Verification items for the finished model (mm, model axes). Face numbers are marked on the shaded views. A direction names the side the tool comes from. Round coordinates to 2 decimals unless told otherwise and drop trailing zeros. Loops run counter-clockwise (first coordinate to the right, second up) from the corner with the lowest first, then second, coordinate; pieces in that order, holes last. Notation, with made-up numbers: M 0,15.5 L 31,15.5 A27 ccw 31,52.5 Z; hole C -18,81 d1. An arc over 180 degrees is marked long. Write item = value, one per line. Start each with the question number.
from build123d import *

# Parameters (mm, degrees)
SKETCH_R     = 4
PAD_DEPTH    = 13
SKETCH001_R  = 2.5
POCKET_DEPTH = 5
FILLET_R     = 14


with BuildPart() as part:
    # Sketch → Pad (new body)
    with BuildSketch(Plane.XY):
        Polygon((27.5, 0), (-27.5, 0), (-27.5, 5), (-14.5, 5), (-14.5, 29), (14.5, 29), (14.5, 5), (27.5, 5), align=None)
        with Locations((0, 14.5)):
            Circle(SKETCH_R, mode=Mode.SUBTRACT)
    extrude(amount=PAD_DEPTH)

    # Sketch001 → Pocket (cut)
    with BuildSketch(Plane.XZ):
        with Locations((-21, 6.5)):
            Circle(SKETCH001_R)
        with Locations((21, 6.5)):
            Circle(SKETCH001_R)
    extrude(amount=-POCKET_DEPTH, mode=Mode.SUBTRACT)

    # Fillet
    fillet_edges = [part.edges().sort_by_distance(p)[0] for p in [
        (-14.5, 29, 6.5),
        (14.5, 29, 6.5),
    ]]
    fillet(fillet_edges, radius=FILLET_R)


solid = part.part
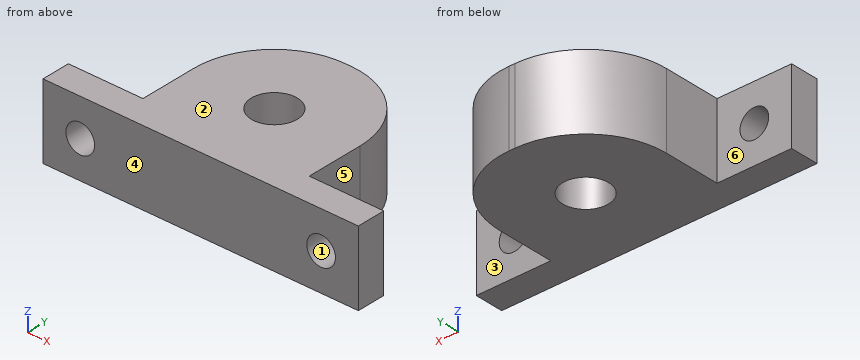
1. Thickness scan on line 1 (X direction, y = 14.25, z = 9.25); line 2 (Z direction, x = 21, y = 2.5); line 3 (Y direction, x = 0, z = 7). Record the ranges inside material, lowest first.
2. Mould release check, pull along Z, two halves, no side actions. Record for the marked faces 1, 2 and 3: pulls with the +Z half, pulls with the -Z half, needs draft (parallel to the pull), parting line crosses it, or undercut.
3. Tool access check on the marked faces 4, 5 and 6. Record the directions out of +Z, -Z, +X, -X, +Y, -Y that give a thin tool (end or side, any length) a straight path to the whole face; none if there is none.
4. Section check B-B, the plane x = 21. Enter the section's corners in (y, z).
5. Gauge pin test, flat ends, axial feed: P1, Ø4.5, axis at x = 21, z = 6.5, coming from the -Y side; P2, Ø1, axis at x = 13.5, z = 9.5, coming from the +Y side; P3, Ø4, axis at y = 24.5, z = 11, coming from the +X side; P4, Ø3, axis at y = 8, z = 3, coming from the +X side. Record the tip position at first contact, or that the pin passes through.
6. Section check D-D, the plane x = 2. Enter the section's corners in (y, z).
7. Section check C-C, the plane x = -16. Enter the section's corners in (y, z), and give its area (3 significant figures).
8. Section check A-A, the plane z = 6.5. Enter the section's corners in (x, y), and give its area (3 significant figures).
Computed values:
q1.line_1 = -14.5 to -3.99, 3.99 to 14.5
q1.line_2 = 0 to 4, 9 to 13
q1.line_3 = 0 to 10.5, 18.5 to 29
q2.face_1 = undercut
q2.face_2 = pulls with the +Z half
q2.face_3 = needs draft
q3.face_4 = +Z, -Z, +X, -X, -Y
q3.face_5 = +Z, -Z, +X, +Y
q3.face_6 = +Z, -Z, -X, +Y
q4.outline = M 0,0 L 5,0 L 5,4 L 0,4 Z; M 0,9 L 5,9 L 5,13 L 0,13 Z
q5.P1 = through
q5.P2 = 21.3
q5.P3 = 12.32
q5.P4 = 14.5
q6.outline = M 0,0 L 11.04,0 L 11.04,13 L 0,13 Z; M 17.96,0 L 28.92,0 L 28.92,13 L 17.96,13 Z
q7.outline = M 0,0 L 5,0 L 5,13 L 0,13 Z
q7.area = 65.0 mm2
q8.outline = M -27.5,0 L -23.5,0 L -23.5,5 L -27.5,5 Z; M -18.5,0 L 18.5,0 L 18.5,5 L 14.5,5 L 14.5,15 A14 ccw 0.5,29 L -0.5,29 A14 ccw -14.5,15 L -14.5,5 L -18.5,5 Z; M 23.5,0 L 27.5,0 L 27.5,5 L 23.5,5 Z; hole C 0,14.5 d8
q8.area = 787 mm2
